Geometry: see drawing. Coordinates: mm, zero at the bounding-box minimum. A direction names the side the tool comes from. Coordinates: 2 decimals unless noted, no trailing zeros. Write each loop counter-clockwise with the first axis right and the second up, starting at its lowest first coordinate (ties: lowest second). Pieces come first, ordered by that corner, then holes.
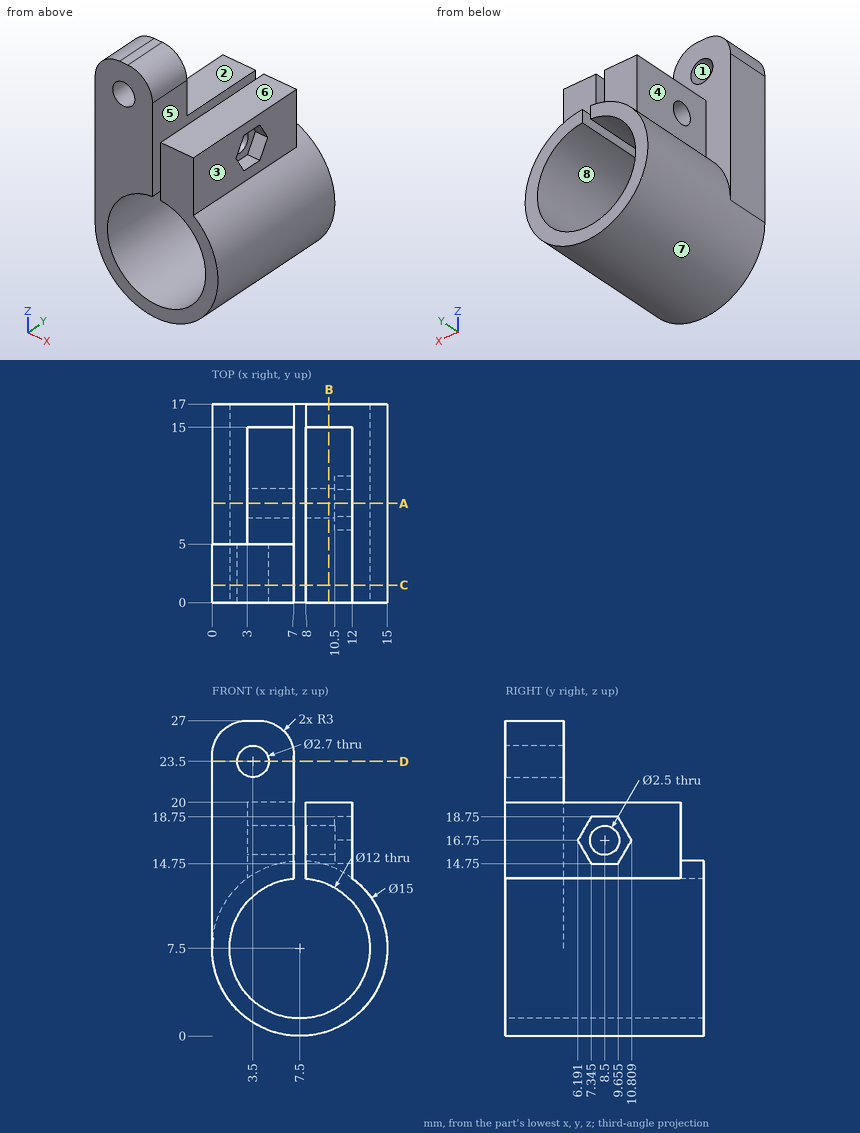
Item 1: Pull-direction query (X, two-part tool) for the marked faces 1, 2, 3 and 4; classes: released by +X, released by -X, zero draft, split by the parting line, or undercut.
Derived:
face 1: undercut
face 2: zero draft
face 3: released by +X
face 4: released by -X
Item 2: Section A-A, the plane y = 8.5. Output: boundary loops of the cut face in (x, z).
Derived:
outline: (3, 13.5) arc R7.5 ccw (long way) to (12, 13.5) - (12, 14.75) - (10.5, 14.75) - (10.5, 15.5) - (8, 15.5) - (8, 13.48) arc R6 cw (long way) to (7, 13.48) - (7, 15.5) - (3, 15.5) - close; (3, 18) - (7, 18) - (7, 20) - (3, 20) - close; (8, 18) - (10.5, 18) - (10.5, 18.75) - (12, 18.75) - (12, 20) - (8, 20) - close
Item 3: Section C-C, the plane y = 1.5. Output: boundary loops of the cut face in (x, z), plus the area to 3 significant figures.
Derived:
outline: (0, 7.5) arc R7.5 ccw (long way) to (12, 13.5) - (12, 20) - (8, 20) - (8, 13.48) arc R6 cw (long way) to (7, 13.48) - (7, 24) arc R3 ccw to (4, 27) - (3, 27) arc R3 ccw to (0, 24) - close; hole circle Ø2.7 at (3.5, 23.5)
area: 171 mm2
Item 4: Material intervals for probe 1 along X at (y, z) = (3.95, 23.5); probe 2 along Z at (x, y) = (7.5, 10); probe 3 along X at (y, z) = (4.25, 2) (1 decimal), sorted ascending.
Derived:
probe 1: x = 0 to 2.15, 4.85 to 7
probe 2: z = 0 to 1.5
probe 3: x = 2.4 to 5.1, 9.9 to 12.6
Item 5: Set-up query: the marked faces 5, 6, 7 and 8. Return all of +Z, -Z, +X, -X, +Y, -Y with unobstructed straight access to the full face (end or side cutting, diameter ignored); none if empty.
Derived:
face 5: +Z, +Y, -Y
face 6: +Z, +X, +Y, -Y
face 7: +Y
face 8: +Y, -Y
Item 6: Section D-D, the plane z = 23.5. Output: boundary loops of the cut face in (x, y).
Derived:
outline: (0, 0) - (2.15, 0) - (2.15, 5) - (0, 5) - close; (4.85, 0) - (7, 0) - (7, 5) - (4.85, 5) - close
Item 7: Pin query (flat end, axial travel): pin 1 (3 mm diameter, centred on y = 8.5, z = 9, fed in from +X); pin 2 (2 mm diameter, centred on y = 11, z = 14, fed in from -X); pin 3 (1.2 mm diameter, centred on x = 5, z = 18, fed in from +Y); pin 4 (2 mm diameter, centred on x = 5, y = 8.5, fed in from +Z). Return the tip coordinate at first contact, or that it passes through.
Derived:
pin 1: stops at x = 15
pin 2: stops at x = 2.4
pin 3: stops at y = 15
pin 4: stops at z = 20
Item 8: Section B-B, the plane x = 10. State how many separate pieces and enclosed holes the cut face has.
Derived:
separate pieces: 2
enclosed holes: 1
